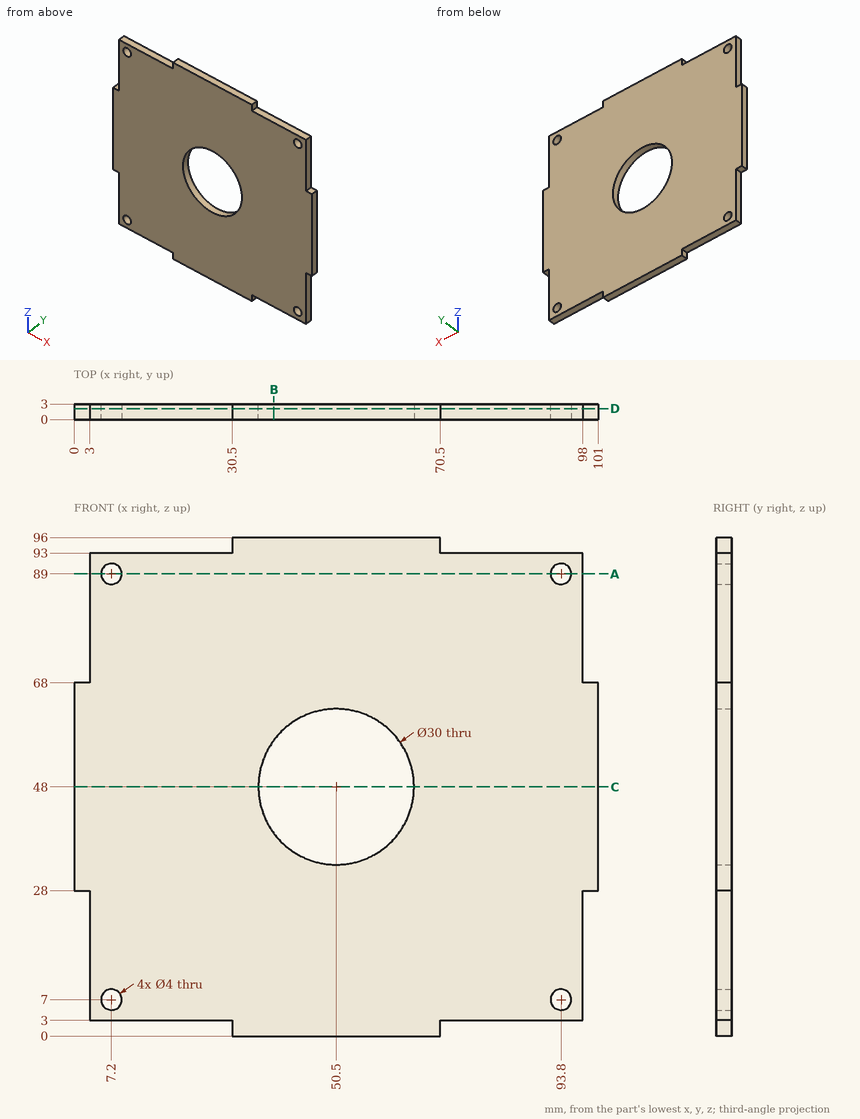
Could you check a few things on this drawing? It's one solid part, dimensions in mm from its lowest x, y, z. Coordinates: 2 decimals unless noted, no trailing zeros. Loops run counter-clockwise (first coordinate to the right, second up) from the corner with the lowest first, then second, coordinate; pieces in that order, holes last. Notation, with made-up numbers: (54.5, 9) - (113.5, 9) arc R26 cw to (113.5, 35) - close; hole circle Ø5 at (40, 26). An arc over 180 degrees is marked (long way). Answer as a JSON object with one key per item and string values. Group by question number.
Item 1: If I drill on L1, parallel to Z at x = 93.8, y = 1.5; L2, parallel to Z at x = 8, y = 1.75; L3, parallel to X at y = 1.95, z = 6.5, over which ranges is the centre line in solid material (lowest first)? Write a range as from..to.
Item 2: If we section it at C-C (z = 48): List the corners of the cut face in (x, y) for me, plus the area to 3 significant figures.
Item 3: If we section it at D-D (y = 2.1): List the corners of the cut face in (x, z) for me.
Item 4: For pin 1 (1.5 mm diameter, centred on y = 2, z = 1, fed in from +X); pin 2 (1 mm diameter, centred on x = 24, y = 1, fed in from -Z); pin 3 (1.5 mm diameter, centred on x = 1, y = 2, fed in from -Z), each with a flat end and sliding along its axis, tell me the tip position at first contact or that it passes through.
Item 5: If we section it at B-B (x = 38.5): List the corners of the cut face in (y, z) for me, plus the area to 3 significant figures.
Item 6: If we section it at A-A (z = 89): List the corners of the cut face in (x, y) for me.
Returned:
{
 "1": {"L1": "z = 3..5, 9..87, 91..93", "L2": "z = 3..5.17, 8.83..87.17, 90.83..93", "L3": "x = 3..5.26, 9.14..91.86, 95.74..98"},
 "2": {"outline": "(0, 0) - (35.5, 0) - (35.5, 3) - (0, 3) - close; (65.5, 0) - (101, 0) - (101, 3) - (65.5, 3) - close", "area": "213 mm²"},
 "3": {"outline": "(0, 28) - (3, 28) - (3, 3) - (30.5, 3) - (30.5, 0) - (70.5, 0) - (70.5, 3) - (98, 3) - (98, 28) - (101, 28) - (101, 68) - (98, 68) - (98, 93) - (70.5, 93) - (70.5, 96) - (30.5, 96) - (30.5, 93) - (3, 93) - (3, 68) - (0, 68) - close; hole circle Ø4 at (7.2, 7); hole circle Ø4 at (7.2, 89); hole circle Ø30 at (50.5, 48); hole circle Ø4 at (93.8, 7); hole circle Ø4 at (93.8, 89)"},
 "4": {"pin 1": "stops at x = 70.5", "pin 2": "stops at z = 3", "pin 3": "stops at z = 28"},
 "5": {"outline": "(0, 0) - (3, 0) - (3, 39) - (0, 39) - close; (0, 57) - (3, 57) - (3, 96) - (0, 96) - close", "area": "234 mm²"},
 "6": {"outline": "(3, 0) - (5.2, 0) - (5.2, 3) - (3, 3) - close; (9.2, 0) - (91.8, 0) - (91.8, 3) - (9.2, 3) - close; (95.8, 0) - (98, 0) - (98, 3) - (95.8, 3) - close"}
}
